Autodesk Inventor part; units mm, degrees
ref_plane "YZ Plane" through (0, 0, 0) normal (1, 0, 0) x (0, 1, 0)
ref_plane "XZ Plane" through (0, 0, 0) normal (0, 1, 0) x (-1, 0, 0)
ref_plane "XY Plane" through (0, 0, 0) normal (0, 0, 1) x (1, 0, 0)
sketch "Szkic1" plane through (0, 0, 0) normal (0, 1, 0) x (-1, 0, 0)
  line L0 (6.65, 5.25) -> (-6.65, 5.25)
  line L1 (-6.65, 5.25) -> (-6.65, -5.25)
  line L2 (-6.65, -5.25) -> (6.65, -5.25)
  line L3 (6.65, -5.25) -> (6.65, 5.25)
  point P0 (0, 0)
  dimension "d0" = 10.5
  dimension "d1" = 5.25
  dimension "d2" = 6.65
  dimension "d3" = 13.3
extrude "Wyciągnięcie proste1" add sketch "Szkic1" along normal blind 1
sketch "Szkic2" plane through (0, 1, 0) normal (0, 1, 0) x (1, 0, 0)
  line L0 (-4.3267, -2.2) -> (-1.9267, -2.2)
  line L1 (-1.9267, -2.2) -> (-1.9267, 2.2)
  line L2 (-1.9267, 2.2) -> (-4.3267, 2.2)
  line L3 (-4.3267, 2.2) -> (-4.3267, -2.2)
  point P0 (0, 0)
  dimension "d6" = 4.4
  dimension "d7" = 2.4
  dimension "d8" = 2.2
extrude "Wyciągnięcie proste2" add sketch "Szkic2" along normal blind 1
properties part number "vl"
The listing builds one solid part. Answer for the finished solid, in the listing's coordinates (mm). A direction names the side the tool comes from. Coordinates: 2 decimals unless noted, no trailing zeros. Write each loop counter-clockwise with the first axis right and the second up, starting at its lowest first coordinate (ties: lowest second). Pieces come first, ordered by that corner, then holes. Notation, with made-up numbers: (68, 8.5) -> (109, 8.5) arc R9 ccw to (109, 24.5) -> close; hole circle Ø7 at (20.5, -34.75). An arc over 180 degrees is marked (long way). Write each question's results on one line, items separated by ' | '. Start each with the question number.
1) A cutting plane is placed at B-B (x = -3.5). Determine the outline of the cut face in (y, z), then the cut area to 3 significant figures.
2) A cutting plane is placed at D-D (x = 2.75). Determine the outline of the cut face in (y, z).
3) Flat-ended cylindrical pins translate along their axes: pin 1 Ø1 at (x, z) = (5.5, -2) entering from +Y; pin 2 Ø0.8 at (y, z) = (1.5, 0.5) entering from -X. Find the tip coordinate at first contact, or state that the pin passes through.
4) A tool of negligible diameter and unlimited length cuts with its end or side. For faces 1 (the flat face through (-4.327, 1.5, 0)), 2 (the flat face through (-3.1, 1.5, -2.2)), 3 (the flat face through (-1.927, 1.5, 0)), from which of +Z, -Z, +X, -X, +Y, -Y can it reach the whole face along a straight path? Write none if from no direction.
5) A cutting plane is placed at C-C (y = 1.6). Determine the outline of the cut face in (x, z), then the cut area to 3 significant figures.
6) A cutting plane is placed at A-A (z = 2). Determine the outline of the cut face in (x, y).
7) Straight lines are drawn through the part: probe 1 along Y at (x, z) = (2.5, 3.5); probe 2 along X at (y, z) = (1.1, -1.75). For each, find the intervals that lie inside material, in ascending order.
Values follow:
1) outline: (0, -5.25) -> (1, -5.25) -> (1, -2.2) -> (2, -2.2) -> (2, 2.2) -> (1, 2.2) -> (1, 5.25) -> (0, 5.25) -> close | area: 14.9 mm²
2) outline: (0, -5.25) -> (1, -5.25) -> (1, 5.25) -> (0, 5.25) -> close
3) pin 1: y = 1 | pin 2: x = -4.33
4) face 1: +Z, -Z, -X, +Y | face 2: -Z, +X, -X, +Y | face 3: +Z, -Z, +X, +Y
5) outline: (-4.33, -2.2) -> (-1.93, -2.2) -> (-1.93, 2.2) -> (-4.33, 2.2) -> close | area: 10.6 mm²
6) outline: (-6.65, 0) -> (6.65, 0) -> (6.65, 1) -> (-1.93, 1) -> (-1.93, 2) -> (-4.33, 2) -> (-4.33, 1) -> (-6.65, 1) -> close
7) probe 1: 0 to 1 | probe 2: -4.33 to -1.93
